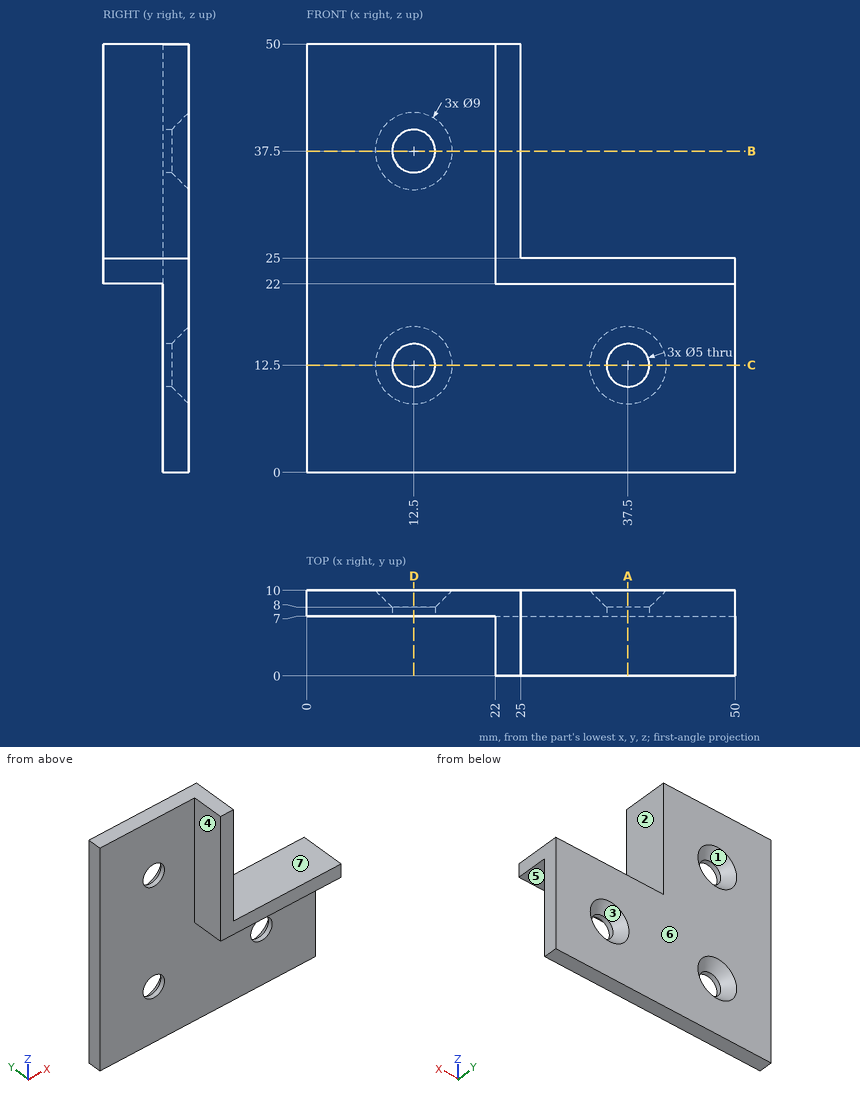
Could you check a few things on this drawing? It's one solid part, dimensions in mm from its lowest x, y, z. A direction names the side the tool comes from. Coordinates: 2 decimals unless noted, no trailing zeros. Loops run counter-clockwise (first coordinate to the right, second up) from the corner with the lowest first, then second, coordinate; pieces in that order, holes last. Notation, with made-up numbers: (4, -13.5) - (53, -13.5) arc R28 ccw to (53, 13.5) - close; hole circle Ø5 at (-8.75, 55.5). An arc over 180 degrees is marked (long way). Answer as a JSON object with one key per item and string values. Group by question number.
Item 1: If we section it at D-D (x = 12.5): List the corners of the cut face in (y, z) for me.
Item 2: If we section it at C-C (z = 12.5): List the corners of the cut face in (x, y) for me.
Item 3: If we section it at A-A (x = 37.5): List the corners of the cut face in (y, z) for me.
Item 4: If I drill on L1, parallel to Z at x = 12.5, y = 7.5; L2, parallel to X at y = 9.75, z = 11, over which ranges is the centre line in solid material (lowest first)? Write a range as from..to.
Item 5: On a 3-axis mill with a long thin cutter (end or side, diameter ignored), from which of +Z, -Z, +X, -X, +Y, -Y can I reach the whole of each face in a straight line? I mean the marked faces 5, 6 and 7. Say none if no direction works.
Item 6: If we section it at B-B (z = 37.5): List the corners of the cut face in (x, y) for me.
Item 7: If we mould it in two halves opening along X, with no side actions, what happens to the marked faces 1, 2, 3 and 4? For each: released by +X, released by -X, zero draft, split by the parting line, or undercut.
Item 8: For pin 1 (3.5 mm diameter, centred on y = 3.5, z = 40, fed in from -X); pin 2 (8 mm diameter, centred on x = 37.5, z = 12.5, fed in from -Y); pin 3 (6 mm diameter, centred on x = 37.5, y = 8, fed in from +Z); pin 4 (25 mm diameter, centred on x = 24.5, z = 15, fed in from -Y), each with a flat end and sliding along its axis, tell me the tip position at first contact or that it passes through.
Returned:
{
 "1": {"outline": "(7, 0) - (10, 0) - (10, 8) - (8, 10) - (7, 10) - close; (7, 15) - (8, 15) - (10, 17) - (10, 33) - (8, 35) - (7, 35) - close; (7, 40) - (8, 40) - (10, 42) - (10, 50) - (7, 50) - close"},
 "2": {"outline": "(0, 7) - (10, 7) - (10, 8) - (8, 10) - (0, 10) - close; (15, 7) - (35, 7) - (35, 8) - (33, 10) - (17, 10) - (15, 8) - close; (40, 7) - (50, 7) - (50, 10) - (42, 10) - (40, 8) - close"},
 "3": {"outline": "(0, 22) - (7, 22) - (7, 15) - (8, 15) - (10, 17) - (10, 25) - (0, 25) - close; (7, 0) - (10, 0) - (10, 8) - (8, 10) - (7, 10) - close"},
 "4": {"L1": "z = 0..10, 15..35, 40..50", "L2": "x = 0..8.52, 16.48..33.52, 41.48..50"},
 "5": {"face 5": "-Z, +X, -X, -Y", "face 6": "+Z, -Z, +X, -X, +Y", "face 7": "+Z, +X, +Y, -Y"},
 "6": {"outline": "(0, 7) - (10, 7) - (10, 8) - (8, 10) - (0, 10) - close; (15, 7) - (22, 7) - (22, 0) - (25, 0) - (25, 10) - (17, 10) - (15, 8) - close"},
 "7": {"face 1": "undercut", "face 2": "released by +X", "face 3": "undercut", "face 4": "released by -X"},
 "8": {"pin 1": "stops at x = 22", "pin 2": "stops at y = 7", "pin 3": "stops at z = 25", "pin 4": "stops at y = 0"}
}
